Autodesk Inventor part; units mm, degrees
ref_plane "Plano de trabajo8" through (0, 0, 79.05) normal (0, 0, 1) x (1, 0, 0)
ref_plane "YZ Plane" through (0, 0, 0) normal (1, 0, 0) x (0, 1, 0)
ref_plane "XZ Plane" through (0, 0, 0) normal (0, 1, 0) x (-1, 0, 0)
sketch "Boceto1" plane through (0, 0, 0) normal (1, 0, 0) x (0, 1, 0)
  point P0 (0, 0)
sketch "Boceto2" plane through (0, 0, 0) normal (1, 0, 0) x (0, 1, 0)
  point P0 (0, 0)
  point P1 (0, 0)
ref_plane "Plano de trabajo1" through (0, 0, 19.45) normal (0, 0, 1) x (1, 0, 0)
sketch "Boceto3" plane through (0, 0, 19.45) normal (0, 0, 1) x (1, 0, 0)
  circle A0 centre (0, 0) radius 5.825
  dimension "d1" = 11.65
ref_plane "Plano de trabajo3" through (0, 0, 62.35) normal (0, 0, 1) x (1, 0, 0)
ref_plane "Plano de trabajo2" through (0, 0, 41) normal (0, 0, 1) x (1, 0, 0)
sketch "Boceto4" plane through (0, 0, 19.45) normal (0, 0, 1) x (1, 0, 0)
  circle A0 centre (0, 0) radius 9.225
  dimension "d4" = 18.45
sketch "Boceto5" plane through (0, 0, 41) normal (0, 0, 1) x (1, 0, 0)
  circle A0 centre (0, 0) radius 4.8
  dimension "d5" = 9.6
sketch "Boceto6" plane through (0, 0, 62.35) normal (0, 0, 1) x (1, 0, 0)
  circle A0 centre (0, 0) radius 9.175
  dimension "d6" = 18.35
ref_plane "Plano de trabajo4" through (0, 0, 66.55) normal (0, 0, 1) x (1, 0, 0)
sketch "Boceto7" plane through (0, 0, 66.55) normal (0, 0, 1) x (1, 0, 0)
  point P0 (0, 0)
sketch "Boceto8" plane through (0, 0, 66.55) normal (0, 0, 1) x (1, 0, 0)
  circle A0 centre (0, 0) radius 3.225
  dimension "d8" = 6.45
ref_plane "Plano de trabajo5" through (0, 0, 70.4) normal (0, 0, 1) x (1, 0, 0)
sketch "Boceto9" plane through (0, 0, 70.4) normal (0, 0, 1) x (1, 0, 0)
  circle A0 centre (0, 0) radius 3.225
  dimension "d10" = 6.45
loft "Solevación1" add profiles "Boceto3" section 1 point at (0, 0, 0)
loft "Solevación2" add profiles "Boceto4", "Boceto5"
loft "Solevación3" add profiles "Boceto6" section 1 edges at (-4.8, 0, 41)
loft "Solevación4" add profiles "Boceto8" section 1 edges at (-9.175, 0, 62.35)
loft "Solevación5" add profiles "Boceto9" section 1 edges at (-3.225, 0, 66.55)
ref_plane "Plano de trabajo8" through (0, 0, 79.05) normal (0, 0, 1) x (1, 0, 0)
ref_plane "Plano de trabajo7" through (0, 0, 76.75) normal (0, 0, 1) x (1, 0, 0)
sketch "Boceto10" plane through (0, 0, 72.75) normal (0, 0, 1) x (1, 0, 0)
  circle A0 centre (0, 0) radius 6.25
  dimension "d34" = 12.5
sketch "Boceto11" plane through (0, 0, 76.75) normal (0, 0, 1) x (1, 0, 0)
  circle A0 centre (0, 0) radius 6.25
  dimension "d35" = 12.5
sketch "Boceto12" plane through (0, 0, 79.05) normal (0, 0, 1) x (1, 0, 0)
  point P0 (0, 0)
sketch "Boceto13" plane through (0, 0, 79.05) normal (0, 0, 1) x (1, 0, 0)
  circle A0 centre (0, 0) radius 3.225
  dimension "d36" = 6.45
loft "Solevación6" add profiles "Boceto10" section 1 edges at (-3.225, 0, 70.4)
loft "Solevación7" add profiles "Boceto11" section 1 edges at (-6.25, 0, 72.75)
loft "Solevación8" add profiles "Boceto13" section 1 edges at (-6.25, 0, 76.75)
sketch "Boceto14" plane through (0, 0, 79.05) normal (0, 0, 1) x (1, 0, 0)
  circle A0 centre (0, 0) radius 1.7
  dimension "d49" = 3.4
extrude "Extrusión1" cut sketch "Boceto14" against normal blind 2.75
sketch "Sketch15" plane through (0, 0, 0) normal (1, 0, 0) x (0, 1, 0)
  circle A0 centre (0, 60.5) radius 1.59
  point P0 (0, 0)
  dimension "d52" = 3.18
  dimension "d53" = 60.5
extrude "Extrusion2" cut sketch "Sketch15" along normal through all both and the other way through all
ref_plane "Plano de trabajo6" through (0, 0, 72.75) normal (0, 0, 1) x (1, 0, 0)
properties part number "BAILARINA"
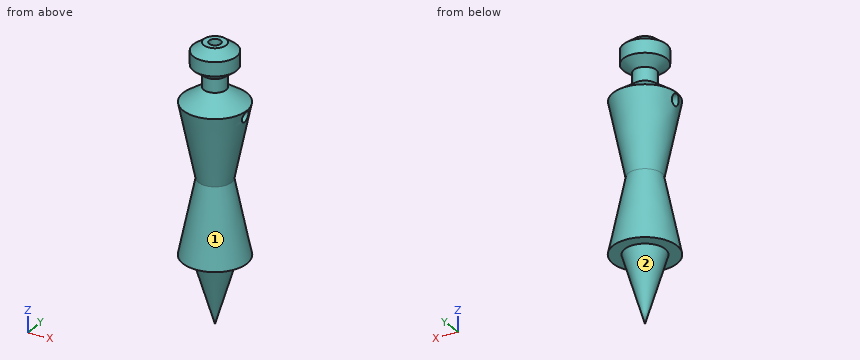
Work out the finished part from the listing and answer in its coordinate system (mm). Face numbers are marked on the shaded views. Coordinates: 2 decimals unless noted, no trailing zeros. Loops run counter-clockwise (first coordinate to the right, second up) from the corner with the lowest first, then second, coordinate; pieces in that order, holes last. Notation, with made-up numbers: (-3.75, 49.5) -> (6.25, 49.5) arc R19 ccw to (6.25, 73.5) -> close; hole circle Ø9 at (73, 79). An arc over 180 degrees is marked (long way). Write each question's results on one line, items separated by ' | '. Start each with the question number.
1) Consider line 1 along Y through (x, z) = (2.25, 50); line 2 along Y through (x, z) = (-1, 60.5); line 3 along Y through (x, z) = (0, 77.55). Determine where each line is inside the solid, lowest interval first.
2) Flat-ended cylindrical pins translate along their axes: P1, Ø1.5, axis at y = -4.5, z = 52, coming from the +X side; P2, Ø4, axis at y = 0, z = 60.5, coming from the -X side (3 decimals); P3, Ø5, axis at x = 3.5, z = 50.5, coming from the -Y side. Find the tip coordinate at first contact, or state that the pin passes through.
3) Find section B-B on z = 60.5. Determine the outline of the cut face in (x, y).
4) The mould has two halves that part along Z. Classify the marked faces 1 and 2: pulls with the +Z half, pulls with the -Z half, needs draft (parallel to the pull), parting line crosses it, or undercut.
5) Find section D-D on z = 17.5. Determine the outline of the cut face in (x, y).
6) Find section A-A on x = -4.5. Count the separate pieces of the cut face and the enclosed holes in it, then the cut area to 3 significant figures.
Response values:
1) line 1: y = -6.25 to 6.25 | line 2: y = -8.74 to -1.59, 1.59 to 8.74 | line 3: y = -5.2 to -1.7, 1.7 to 5.2
2) P1: stops at x = 6.01 | P2: stops at x = -9.175 | P3: stops at y = -6.9
3) outline: (-8.65, -1.59) arc R8.8 ccw to (8.65, -1.59) -> close; (-8.65, 1.59) -> (8.65, 1.59) arc R8.8 ccw to start
4) face 1: undercut | face 2: pulls with the -Z half
5) outline: circle Ø10.48 at (0, 0)
6) separate pieces: 2 | enclosed holes: 1 | area: 544 mm^2
